```python
from build123d import *

# Parameters (mm, degrees)
SKETCH1_R             = 5.75
BOSS_EXTRUDE1_DEPTH   = 3
BOSS_EXTRUDE2_DEPTH   = 0.3
CIRPATTERN1_COUNT     = 2
SKETCH4_R             = 2.5
CUT_EXTRUDE1_DEPTH    = 16.3
CHAMFER1_SIZE         = 1
CHAMFER1_SIZE2        = 1.191753593
CHAMFER1_PART_2_SIZE  = 1
CHAMFER1_PART_2_SIZE2 = 1.191753593


with BuildPart() as part:
    # Sketch1 → Boss-Extrude1 (new body, symmetric)
    with BuildSketch(Plane(origin=(0, 0, 0), x_dir=(1, 0, 0), z_dir=(0, 1, 0))):
        Circle(SKETCH1_R)
    extrude(amount=BOSS_EXTRUDE1_DEPTH, both=True)

    # Sketch3 → Boss-Extrude2 (add)
    with BuildSketch(Plane(origin=(0, 0, 0), x_dir=(0.974370065, -0.224951054, 0), z_dir=(-0.224951054, -0.974370065, 0))):
        with BuildLine():
            Line((-6.906213286, 5.083465827), (-4.318560917, 2.607550724))
            Line((-4.318560917, 2.607550724), (5.113121785, 2.549410262))
            add(Edge.make_bspline(
                [(5.113121785, 2.549410262), (5.735638165, 8.028953924), (4.346346729, 38.97674066), (0.38313372, 57.205124306), (0.080525316, 59.236652626)],
                knots=[0, 0, 0, 0, 0.55249972, 0.930981027, 0.930981027, 0.930981027, 0.930981027], degree=3))
            ThreePointArc((0.080525316, 59.236652626), (-1.600195584, 62.287034666), (-4.864911258, 63.5))
            Line((-4.864911258, 63.5), (-5.4532168, 63.5))
            ThreePointArc((-5.4532168, 63.5), (-6.874270643, 62.907340035), (-7.453122766, 61.480605975))
            Line((-7.453122766, 61.480605975), (-6.906213286, 5.083465827))
        make_face()
    boss_extrude2 = extrude(amount=BOSS_EXTRUDE2_DEPTH)

    # CirPattern1: Boss-Extrude2 ×2 about axis
    cirpattern1_axis = Axis((0, -3, 0), (0, 1, 0))
    for i in range(1, CIRPATTERN1_COUNT):
        add(boss_extrude2.rotate(cirpattern1_axis, i * 360 / CIRPATTERN1_COUNT))

    # Sketch4 → Cut-Extrude1 (cut)
    with BuildSketch(Plane.XZ.offset(3)):
        Circle(SKETCH4_R)
    extrude(amount=-CUT_EXTRUDE1_DEPTH, mode=Mode.SUBTRACT)

    # Chamfer1
    chamfer1_edges = [part.edges().sort_by_distance(p)[0] for p in [
        (-2.5, 3, 0),
    ]]
    chamfer1_side = [part.faces().sort_by_distance(p)[0] for p in [
        (-5.58736544, 3, 0),
    ]]
    chamfer(chamfer1_edges, length=CHAMFER1_SIZE, length2=CHAMFER1_SIZE2, reference=chamfer1_side[0])

    # Chamfer1 part 2
    chamfer1_part_2_edges = [part.edges().sort_by_distance(p)[0] for p in [
        (-2.5, -3, 0),
    ]]
    chamfer1_part_2_side = [part.faces().sort_by_distance(p)[0] for p in [
        (-5.58736544, -3, 0),
    ]]
    chamfer(chamfer1_part_2_edges, length=CHAMFER1_PART_2_SIZE, length2=CHAMFER1_PART_2_SIZE2, reference=chamfer1_part_2_side[0])


solid = part.part
```
Model file for the job. Use its own axes, mm. A direction names the side the tool comes from. Coordinates: 2 decimals unless noted, no trailing zeros. Order: outer loops, then holes, each group sorted by start corner. A loop starts at its lowest first (then second) coordinate and runs counter-clockwise, first axis right, second up. Notation, with made-up numbers: (81.25, 9.25) - (105.25, 9.25) arc R18 cw to (105.25, 34.25) - close; hole circle Ø6 at (45, 30.25). An arc over 180 degrees is marked (long way). Return JSON: item names as keys, results as strings. Group by question number.
1) Probe line 1 (Z direction, x = 0, y = 0.25); line 2 (Z direction, x = 0.75, y = -2.5); line 3 (Z direction, x = 5, y = 0.75). List the from-to ranges inside material, lowest first. Write a range as from..to.
2) Flat gauge pins, fed straight in: P1, Ø1, axis at x = 0, y = 1.5, coming from the +Z side; P2, Ø1.5, axis at x = -5.5, y = 1.5, coming from the -Z side; P3, Ø1.5, axis at x = 2, y = -1.5, coming from the -Z side. Where does each tip first touch, or does it go through?
3) Saw through at A-A, the plane z = 0. Write the cut outline in (x, y), plus the area to 3 significant figures.
4) Tool access for faces 1 (the cylindrical face through (-4.238, 0.042, -3.886)), 2 (the flat face through (0, -3, 4)): list every direction of +Z, -Z, +X, -X, +Y, -Y with a clear straight run to the whole face (end or side of a thin tool).
5) Mould opens along X. For faces 3 (the flat face through (0, 3, 4)), 4 (the cylindrical face through (-0.54, -0.03, -2.44)) say: released by +X, released by -X, zero draft, split by the parting line, or undercut.
Values found:
{
 "1": {"line 1": "z = -5.75..-2.5, 2.5..5.75", "line 2": "z = -5.7..-2.99, 2.99..5.7", "line 3": "z = -2.84..2.84"},
 "2": {"P1": "stops at z = 5.75", "P2": "stops at z = -3.24", "P3": "stops at z = -5.61"},
 "3": {"outline": "(-5.75, -3) - (-3.5, -3) - (-2.5, -1.81) - (-2.5, 1.81) - (-3.5, 3) - (-5.75, 3) - close; (2.5, -1.81) - (3.5, -3) - (5.75, -3) - (5.75, 3) - (3.5, 3) - (2.5, 1.81) - close", "area": "36.6 mm²"},
 "4": {"face 1": "none", "face 2": "+Z, -Z, +X, -X, -Y"},
 "5": {"face 3": "zero draft", "face 4": "undercut"}
}
